Model file for the job. Use its own axes, mm. A direction names the side the tool comes from. Give positions to 0.01 mm unless a question says otherwise; leave off trailing zeros. Loops run counter-clockwise (first coordinate to the right, second up) from the corner with the lowest first, then second, coordinate; pieces in that order, holes last. Notation, with made-up numbers: (-34.75, -6) - (-19.75, -6) arc R26 ccw to (-19.75, 23) - close; hole circle Ø8 at (44.5, 26.25). An arc over 180 degrees is marked (long way). Use a Markdown table: item, result.
Autodesk Inventor part; units mm, degrees
ref_plane "YZ Plane" through (0, 0, 0) normal (1, 0, 0) x (0, 1, 0)
ref_plane "XZ Plane" through (0, 0, 0) normal (0, 1, 0) x (-1, 0, 0)
ref_plane "XY Plane" through (0, 0, 0) normal (0, 0, 1) x (1, 0, 0)
sketch "Sketch2" plane through (0, 0, 0) normal (0, 1, 0) x (-1, 0, 0)
  line L0 (16, -6.6684) -> (16, 6.6684)
  line L1 (9.675, -1.4184) -> (12.925, -1.4184)
  line L2 (12.925, -1.4184) -> (12.925, -2.9684)
  line L3 (12.925, -2.9684) -> (4.35, -2.9684)
  line L4 (4.35, -2.9684) -> (4.35, -4.6684)
  line L5 (4.35, -4.6684) -> (-4.35, -4.6684)
  line L6 (-4.35, -4.6684) -> (-4.35, -3.6684)
  line L7 (-9.675, -2.9684) -> (-12.925, -2.9684)
  line L8 (-12.925, -2.9684) -> (-12.925, -1.4184)
  line L9 (-12.925, -1.4184) -> (-9.675, -1.4184)
  line L10 (-9.675, -1.4184) -> (-9.675, 0.5816)
  line L11 (-9.675, 0.5816) -> (-14.925, 0.5816)
  line L12 (-14.925, 0.5816) -> (-14.925, -6.6684)
  line L13 (14.925, -6.6684) -> (14.925, 0.5816)
  line L14 (14.925, 0.5816) -> (9.675, 0.5816)
  line L15 (9.675, 0.5816) -> (9.675, -1.4184)
  line L16 (-9.675, -2.9684) -> (-9.675, -3.6684)
  line L17 (-9.675, -3.6684) -> (-4.35, -3.6684)
  line L18 (-16, -6.6684) -> (16, -6.6684)
  line L19 (0, 0) -> (0, -6.6684) construction
  dimension "d2" = 25.25
  dimension "d5" = 0.95
  dimension "d11" = 0.7
  dimension "d13" = 2
  dimension "d14" = 2
  dimension "d16" = 1.1
  dimension "d22" = 8.1
  dimension "d23" = 3.25
  dimension "d24" = 2
extrude "Extrusion2" add sketch "Sketch2" along normal blind 16
sketch "Sketch4" plane through (0, 16, 0) normal (0, 1, 0) x (1, 0, 0)
  line L0 (-4.35, 4.6684) -> (4.35, 4.6684)
  line L1 (14.925, 6.6684) -> (-14.925, 6.6684)
  line L2 (-4.35, 4.6684) -> (-4.35, 6.6684)
  line L3 (4.35, 4.6684) -> (4.35, 6.6684)
  point P0 (0, 0)
extrude "Extrusion4" cut sketch "Sketch4" against normal blind 6.5
sketch "Sketch5" plane through (0, 0, 0) normal (0, -1, 0) x (1, 0, 0)
  line L0 (-9.675, -1.4184) -> (-12.925, -1.4184)
  line L1 (-9.675, 0.5816) -> (-9.675, -1.4184)
  line L2 (-14.925, 0.5816) -> (-9.675, 0.5816)
  line L3 (-14.925, -6.6684) -> (-14.925, 0.5816)
  line L4 (14.925, -6.6684) -> (-14.925, -6.6684)
  line L5 (14.925, 0.5816) -> (14.925, -6.6684)
  line L6 (9.675, 0.5816) -> (14.925, 0.5816)
  line L7 (9.675, -1.4184) -> (9.675, 0.5816)
  line L8 (12.925, -1.4184) -> (9.675, -1.4184)
  line L9 (12.925, -2.9684) -> (12.925, -1.4184)
  line L10 (9.675, -2.9684) -> (12.925, -2.9684)
  line L11 (9.675, -3.6684) -> (9.675, -2.9684)
  line L12 (4.35, -3.6684) -> (9.675, -3.6684)
  line L13 (4.35, -4.6684) -> (4.35, -3.6684)
  line L14 (-4.35, -4.6684) -> (4.35, -4.6684)
  line L15 (-4.35, -2.9684) -> (-4.35, -4.6684)
  line L16 (-12.925, -2.9684) -> (-4.35, -2.9684)
  line L17 (-12.925, -1.4184) -> (-12.925, -2.9684)
  line L18 (-14.925, 0.5816) -> (-4.55, 8.5816)
  line L19 (-4.55, 8.5816) -> (-4.55, 19.3316)
  line L20 (-4.55, 19.3316) -> (4.55, 19.3316)
  line L21 (4.55, 19.3316) -> (4.55, 8.5816)
  line L22 (4.55, 8.5816) -> (14.925, 0.5816)
  line L23 (0, -6.6684) -> (0, 19.3316) construction
  point P0 (0, 0)
  dimension "d27" = 9.5
  dimension "d28" = 26
  dimension "d29" = 8
extrude "Extrusion5" add sketch "Sketch5" along normal blind 2.75
sketch "Sketch6" plane through (0, 0, 0) normal (0, 1, 0) x (1, 0, 0)
  line L0 (-4.55, -19.3316) -> (-4.55, -8.5816)
  line L1 (4.55, -19.3316) -> (-4.55, -19.3316)
  line L2 (4.55, -8.5816) -> (4.55, -19.3316)
  line L3 (-4.55, -8.5816) -> (-4.55, -6.5316)
  line L4 (-4.55, -6.5316) -> (4.55, -6.5316)
  line L5 (4.55, -6.5316) -> (4.55, -8.5816)
  point P0 (0, 0)
  dimension "d32" = 13.2
extrude "Extrusion6" add sketch "Sketch6" along normal blind 2
fillet "Fillet1" radius 2 4 edges at (-4.55, 1, 6.5316) (4.55, 1, 6.5316) (-4.55, -0.375, 19.3316) (4.55, -0.375, 19.3316)
sketch "Sketch7" plane through (0, 2, 0) normal (0, 1, 0) x (1, 0, 0)
  line L0 (4.55, -17.3316) -> (4.55, -8.5316)
  line L1 (2.55, -6.5316) -> (-2.55, -6.5316)
  line L2 (-4.55, -8.5316) -> (-4.55, -17.3316)
  line L3 (-2.55, -19.3316) -> (2.55, -19.3316)
  line L4 (-4, -11.4316) -> (4, -11.4316)
  line L5 (4, -8.4316) -> (-4, -8.4316)
  line L6 (-4, -14.4316) -> (4, -14.4316)
  line L7 (4, -17.4316) -> (-4, -17.4316)
  line L8 (-4.55, -12.9316) -> (4.55, -12.9316) construction
  line L9 (0, -6.5316) -> (0, -19.3316) construction
  line L10 (-4, -8.4316) -> (-4, -11.4316)
  line L11 (-4, -14.4316) -> (-4, -17.4316)
  line L12 (4, -8.4316) -> (4, -11.4316)
  line L13 (4, -14.4316) -> (4, -17.4316)
  point P0 (0, 0)
  dimension "d36" = 3
  dimension "d37" = 3
  dimension "d38" = 3
  dimension "d39" = 8
extrude "Extrusion7" add sketch "Sketch7" along normal blind 5
fillet "Fillet2" radius 3 2 edges at (14.925, 6.625, -6.6684) (-14.925, 6.625, -6.6684)
equation "\"d13\" = d14"
properties part number "PiCam Holder"
(1) 3-axis set-ups, long thin cutter, end or side, ignore diameter. For faces 4 (the flat face through (9.675, 8, 0)), 5 (the flat face through (-4, 4, 10)), 6 (the flat face through (0, 9.5, -6)), 7 (the flat face through (0, 5, -4.668)): which of +Z, -Z, +X, -X, +Y, -Y reach the whole face in a straight line?
Computed:
| item | result |
|---|---|
| face 4 | +Z, +Y |
| face 5 | +Z, -X, +Y |
| face 6 | +Z, -Z, +Y |
| face 7 | +Y |
(2) Slice it at B-B, the plane y = 14. Write the cut outline in (x, z) (3 decimals), plus the area to 3 significant figures.
Computed:
| item | result |
|---|---|
| outline | (-14.925, -3.668) arc R3 ccw to (-11.925, -6.668) - (-4.35, -6.668) - (-4.35, -2.968) - (-12.925, -2.968) - (-12.925, -1.418) - (-9.675, -1.418) - (-9.675, 0.582) - (-14.925, 0.582) - close; (4.35, -6.668) - (11.925, -6.668) arc R3 ccw to (14.925, -3.668) - (14.925, 0.582) - (9.675, 0.582) - (9.675, -1.418) - (12.925, -1.418) - (12.925, -2.968) - (9.675, -2.968) - (9.675, -3.668) - (4.35, -3.668) - close |
| area | 97.9 mm² |
(3) Slice it at A-A, the plane z = -1. Write the cut outline in (x, y) (3 decimals), plus the area to 3 significant figures.
Computed:
| item | result |
|---|---|
| outline | (-14.925, -2.75) - (14.925, -2.75) - (14.925, 16) - (9.675, 16) - (9.675, 0) - (-9.675, 0) - (-9.675, 16) - (-14.925, 16) - close |
| area | 250 mm² |
(4) Slice it at C-C, the plane x = -1.25. Write the cut outline in (y, z), plus the area to 3 significant figures.
Computed:
| item | result |
|---|---|
| outline | (-2.75, -6.67) - (9.5, -6.67) - (9.5, -4.67) - (0, -4.67) - (0, 6.53) - (2, 6.53) - (2, 8.43) - (7, 8.43) - (7, 11.43) - (2, 11.43) - (2, 14.43) - (7, 14.43) - (7, 17.43) - (2, 17.43) - (2, 19.33) - (-2.75, 19.33) - close |
| area | 146 mm² |
(5) Slice it at D-D, the plane y = 8.5. Write the cut outline in (x, z) (3 decimals), plus the area to 3 significant figures.
Computed:
| item | result |
|---|---|
| outline | (-14.925, -3.668) arc R3 ccw to (-11.925, -6.668) - (11.925, -6.668) arc R3 ccw to (14.925, -3.668) - (14.925, 0.582) - (9.675, 0.582) - (9.675, -1.418) - (12.925, -1.418) - (12.925, -2.968) - (9.675, -2.968) - (9.675, -3.668) - (4.35, -3.668) - (4.35, -4.668) - (-4.35, -4.668) - (-4.35, -2.968) - (-12.925, -2.968) - (-12.925, -1.418) - (-9.675, -1.418) - (-9.675, 0.582) - (-14.925, 0.582) - close |
| area | 115 mm² |
(6) Mould opens along X. For faces 1 (the flat face through (-9, 8, -2.968)), 2 (the flat face through (0, 4, 11.432)), 3 (the flat face through (4.55, 0, 13)) say: pulls with the +X half, pulls with the -X half, needs draft (parallel to the pull), parting line crosses it, or undercut.
Computed:
| item | result |
|---|---|
| face 1 | undercut |
| face 2 | needs draft |
| face 3 | pulls with the +X half |
(7) Pin check, flat tips, straight feed: P1, Ø3.5, axis at y = 4.5, z = 16, coming from the +X side; P2, Ø4, axis at x = 12.5, y = 8.5, coming from the +Z side; P3, Ø2.5, axis at y = 3.5, z = 16, coming from the -X side. Stop position of each tip, or through.
Computed:
| item | result |
|---|---|
| P1 | x = 4 |
| P2 | z = 0.58 |
| P3 | x = -4 |
(8) Drill centre lines: probe 1 along Z at (x, y) = (10.75, 12); probe 2 along X at (y, z) = (0.75, 17); probe 3 along Z at (x, y) = (6, 11.25). Where is each one in solid material? Low to high. Write a range as [from, to].
Computed:
| item | result |
|---|---|
| probe 1 | [-6.67, -2.97], [-1.42, 0.58] |
| probe 2 | [-4.55, 4.55] |
| probe 3 | [-6.67, -3.67] |
